Read the model definition and answer for the solid it produces. Units are mm, in the model's axes. A direction names the side the tool comes from. Round coordinates to 2 decimals unless told otherwise and drop trailing zeros. Order: outer loops, then holes, each group sorted by start corner. A loop starts at its lowest first (then second) coordinate and runs counter-clockwise, first axis right, second up. Notation, with made-up numbers: (66, 7) - (112, 7) arc R37 cw to (112, 44) - close; hole circle Ø1 at (37.25, 59). An arc over 180 degrees is marked (long way). Put each result on its own line as item: value. Start each with the question number.
Q1. Which of the six approach directions +Z, -Z, +X, -X, +Y, -Y give full straight-line access (tool end or side, diameter ignored) to faces 5 (the face through (15, 8.905, 37)), 6 (the face through (-2.42, 9, 33)), 7 (the face through (10.62, 7, 20))?
Q2. Find the intervals of material crossed by line 1 along X through (y, z) = (11.5, 15) (3 decimals); line 2 along X through (y, z) = (8, 34.5) (3 decimals); line 3 along X through (y, z) = (9.5, 20) (3 decimals), in increasing order. Write a range as from..to.
Q3. Section C-C on y = 11.5 is taken. Give the vertices of the cut face in (x, z) (1 decimal).
Q4. For a pull along Y with two mould halves and no side action, classify faces 1 (the face through (2, 12.283, 20)), 2 (the face through (-7.701, 16.119, 0.145)), 3 (the face through (4.08, 18, 17)), 4 (the face through (18.75, -0.26, 7.73)) as pulls with the +Y half, pulls with the -Y half, needs draft (parallel to the pull), parting line crosses it, or undercut.
Q5. Section A-A on x = 0 is taken. Give the vertices of the cut face in (y, z), then the cut area to 3 significant figures.
Q6. Section D-D on y = 17 is taken. State how many separate pieces and enclosed holes the cut face has, then the cut area to 3 significant figures.
Q7. Each of these flat-tipped pins is pushed along its axis until it touches: pin 1 Ø2 at (x, z) = (14.5, 8) entering from +Y; pin 2 Ø3.5 at (y, z) = (7, 16.5) entering from +X (3 decimals); pin 3 Ø4 at (x, y) = (10.5, 6) entering from +Z; pin 4 Ø4 at (x, z) = (0, 19.84) entering from +Y. Where does it stop, or does it pass through?
from build123d import *

# Parameters (mm, degrees)
BOSS_EXTRUDE1_DEPTH = 39.6875
SKETCH3_R           = 1.5875
CUT_EXTRUDE1_DEPTH  = 39.6875
CUT_EXTRUDE3_DEPTH  = 5
CUT_EXTRUDE5_DEPTH  = 6.5
FILLET1_R           = 0.508
SKETCH7_W           = 5.08
SKETCH7_H           = 10.72628101
BOSS_EXTRUDE2_DEPTH = 1.905
SKETCH8_W           = 5.08
SKETCH8_H           = 3.15692897
BOSS_EXTRUDE3_DEPTH = 10.16
CUT_EXTRUDE7_REACH  = 55.172
SKETCH9_R           = 1.143
FILLET2_R           = 0.381


with BuildPart() as part:
    # Sketch2 → Boss-Extrude1 (new body)
    with BuildSketch(Plane.XY):
        Polygon((-5.545, 3.02911179), (-10.62, 3.02911179), (-10.62, 10.33111179), (-2.42, 10.33111179), (-2.42, 7.28311179), (2.42, 7.28311179), (2.42, 10.33111179), (10.62, 10.33111179), (10.62, 3.02911179), (5.545, 3.02911179), (5.545, -1.82088821), (13.795, -1.82088821), (13.795, 13.37911179), (10.695, 13.37911179), (4.8375, 19.15761179), (4.8375, 22.33261179), (3.25, 22.33261179), (3.25, 21.57061179), (-3.25, 21.57061179), (-3.25, 22.33261179), (-4.8375, 22.33261179), (-4.8375, 19.15761179), (-10.695, 13.37911179), (-13.795, 13.37911179), (-13.795, -1.82088821), (-5.545, -1.82088821), align=None)
    extrude(amount=BOSS_EXTRUDE1_DEPTH)

    # Sketch3 → Cut-Extrude1 (cut)
    with BuildSketch(Plane(origin=(0, 21.57061179, 0), x_dir=(1, 0, 0), z_dir=(0, 1, 0))):
        with Locations(Location((0, -19.84375, 0), (0, 0, 270))):
            Circle(SKETCH3_R)
    extrude(amount=-CUT_EXTRUDE1_DEPTH, mode=Mode.SUBTRACT)

    # Sketch4 → Cut-Extrude3 (cut)
    with BuildSketch(Plane.XZ.offset(-7.28311179)):
        Polygon((2.078460969, 16.24375), (4.156921938, 19.84375), (2.078460969, 23.44375), (-2.078460969, 23.44375), (-4.156921938, 19.84375), (-2.078460969, 16.24375), align=None)
    extrude(amount=-CUT_EXTRUDE3_DEPTH, mode=Mode.SUBTRACT)

    # Sketch5 → Cut-Extrude5 (cut)
    with BuildSketch(Plane.ZY.offset(2.42)):
        with BuildLine():
            Line((30.935486639, 21.929608435), (6.793752093, 21.929608435))
            ThreePointArc((6.793752093, 21.929608435), (14.106882481, 15.699384594), (9.473965766, 7.28311179))
            Line((9.473965766, 7.28311179), (17.626036587, 7.28311179))
            Line((17.626036587, 7.28311179), (17.626036587, 21.128362833))
            Line((17.626036587, 21.128362833), (21.966828552, 21.128362833))
            Line((21.966828552, 21.128362833), (21.966828552, 7.28311179))
            Line((21.966828552, 7.28311179), (30.118899373, 7.28311179))
            ThreePointArc((30.118899373, 7.28311179), (24.926702023, 14.918604722), (30.935486639, 21.929608435))
        make_face()
    extrude(amount=-CUT_EXTRUDE5_DEPTH, mode=Mode.SUBTRACT)

    # Fillet1
    fillet1_edges = [part.edges().sort_by_distance(p)[0] for p in [
        (-13.795, 5.77911179, 39.6875),
        (-9.67, -1.82088821, 39.6875),
        (-10.62, 6.68011179, 39.6875),
        (-6.52, 10.33111179, 39.6875),
        (-2.42, 8.80711179, 39.6875),
        (-9.67, -1.82088821, 0),
        (0, 7.28311179, 39.6875),
        (-13.795, 5.77911179, 0),
        (-12.245, 13.37911179, 0),
        (-7.76625, 16.26836179, 0),
        (-4.8375, 20.74511179, 0),
        (-4.04375, 22.33261179, 0),
        (-3.25, 21.95161179, 0),
        (0, 21.57061179, 0),
        (3.25, 21.95161179, 0),
        (4.04375, 22.33261179, 0),
        (4.8375, 20.74511179, 0),
        (2.42, 8.80711179, 39.6875),
        (7.76625, 16.26836179, 0),
        (12.245, 13.37911179, 0),
        (13.795, 5.77911179, 0),
        (9.67, -1.82088821, 0),
        (5.545, 0.60411179, 0),
        (8.0825, 3.02911179, 0),
        (10.62, 6.68011179, 0),
        (6.52, 10.33111179, 0),
        (2.42, 8.80711179, 0),
        (0, 7.28311179, 0),
        (6.52, 10.33111179, 39.6875),
        (-2.42, 8.80711179, 0),
        (-6.52, 10.33111179, 0),
        (-10.62, 6.68011179, 0),
        (-8.0825, 3.02911179, 0),
        (-5.545, 0.60411179, 0),
        (10.62, 6.68011179, 39.6875),
        (8.0825, 3.02911179, 39.6875),
        (5.545, 0.60411179, 39.6875),
        (9.67, -1.82088821, 39.6875),
        (-5.545, 0.60411179, 39.6875),
        (13.795, 5.77911179, 39.6875),
        (12.245, 13.37911179, 39.6875),
        (7.76625, 16.26836179, 39.6875),
        (4.8375, 20.74511179, 39.6875),
        (4.04375, 22.33261179, 39.6875),
        (3.25, 21.95161179, 39.6875),
        (0, 21.57061179, 39.6875),
        (-3.25, 21.95161179, 39.6875),
        (-4.04375, 22.33261179, 39.6875),
        (-4.8375, 20.74511179, 39.6875),
        (-8.0825, 3.02911179, 39.6875),
        (-7.76625, 16.26836179, 39.6875),
        (-12.245, 13.37911179, 39.6875),
    ]]
    fillet(fillet1_edges, radius=FILLET1_R)

    # Sketch7 → Boss-Extrude2 (add)
    with BuildSketch(Plane(origin=(13.795, 0, 0), x_dir=(0, 0, -1), z_dir=(1, 0, 0))):
        with Locations((-36.6395, 3.542252295)):
            Rectangle(SKETCH7_W, SKETCH7_H)
        with Locations((-7.4295, 3.542252295)):
            Rectangle(SKETCH7_W, SKETCH7_H)
    extrude(amount=BOSS_EXTRUDE2_DEPTH)

    # Sketch8 → Boss-Extrude3 (add)
    with BuildSketch(Plane(origin=(15.7, 0, 0), x_dir=(0, 0, -1), z_dir=(1, 0, 0))):
        with Locations((-36.6395, -0.242423725)):
            Rectangle(SKETCH8_W, SKETCH8_H)
        with Locations((-7.4295, -0.242423725)):
            Rectangle(SKETCH8_W, SKETCH8_H)
    extrude(amount=BOSS_EXTRUDE3_DEPTH)

    # Sketch9 → Cut-Extrude7 (cut, up to next)
    with BuildSketch(Plane.XZ.offset(1.82088821), mode=Mode.PRIVATE) as cut_extrude7_sk1:
        with Locations((19.891, 35.8775)):
            Circle(SKETCH9_R)
    cut_extrude7_tool1 = extrude(cut_extrude7_sk1.sketch, amount=-CUT_EXTRUDE7_REACH, mode=Mode.PRIVATE) & part.part
    # Sketch9 → Cut-Extrude7 (cut, up to next)
    with BuildSketch(Plane.XZ.offset(1.82088821), mode=Mode.PRIVATE) as cut_extrude7_sk2:
        with Locations((19.891, 7.6835)):
            Circle(SKETCH9_R)
    cut_extrude7_tool2 = extrude(cut_extrude7_sk2.sketch, amount=-CUT_EXTRUDE7_REACH, mode=Mode.PRIVATE) & part.part
    add(cut_extrude7_tool1.solids().sort_by_distance((19.891, -1.820888, 35.8775))[0], mode=Mode.SUBTRACT)
    add(cut_extrude7_tool2.solids().sort_by_distance((19.891, -1.820888, 7.6835))[0], mode=Mode.SUBTRACT)

    # Fillet2
    fillet2_edges = [part.edges().sort_by_distance(p)[0] for p in [
        (18.748, 1.33604076, 35.8775),
        (18.748, -1.82088821, 35.8775),
        (18.748, 1.33604076, 7.6835),
        (18.748, -1.82088821, 7.6835),
    ]]
    fillet(fillet2_edges, radius=FILLET2_R)


solid = part.part
Findings:
1. face 5: +Z, -Z, +X, +Y
1. face 6: +Z, -Z, -Y
1. face 7: +Z, -Z
2. line 1: -13.795..-2.42, 4.08..13.795
2. line 2: -13.795..-10.62, -2.42..2.42, 10.62..15.7
2. line 3: -13.795..-10.62, 10.62..13.795
3. outline: (-13.8, 0.5) arc R0.5 ccw to (-13.3, 0) - (13.3, 0) arc R0.5 ccw to (13.8, 0.5) - (13.8, 39.2) arc R0.5 ccw to (13.3, 39.7) - (-13.3, 39.7) arc R0.5 ccw to (-13.8, 39.2) - close; hole (-4.2, 19.8) - (-2.4, 16.8) - (-2.4, 13.7) - (4.1, 13.7) - (4.1, 17.6) - (2.9, 17.6) - (4.2, 19.8) - (2.9, 22) - (4.1, 22) - (4.1, 25.5) - (-2.4, 25.5) - (-2.4, 22.9) - close
4. face 1: pulls with the -Y half
4. face 2: pulls with the +Y half
4. face 3: undercut
4. face 4: needs draft
5. outline: (7.28, 0.51) arc R0.51 ccw to (7.79, 0) - (21.06, 0) arc R0.51 ccw to (21.57, 0.51) - (21.57, 8.94) arc R7.6 ccw to (7.28, 9.47) - close; (7.28, 30.12) arc R7.6 ccw to (21.57, 29.74) - (21.57, 39.18) arc R0.51 ccw to (21.06, 39.69) - (7.79, 39.69) arc R0.51 ccw to (7.28, 39.18) - close; (12.28, 17.63) - (21.13, 17.63) - (21.13, 18.26) - (12.28, 18.26) - close; (12.28, 21.43) - (21.13, 21.43) - (21.13, 21.97) - (12.28, 21.97) - close
5. area: 386 mm2
6. separate pieces: 1
6. enclosed holes: 3
6. area: 502 mm2
7. pin 1: y = 13.38
7. pin 2: x = 13.795
7. pin 3: z = 39.69
7. pin 4: y = 21.13
